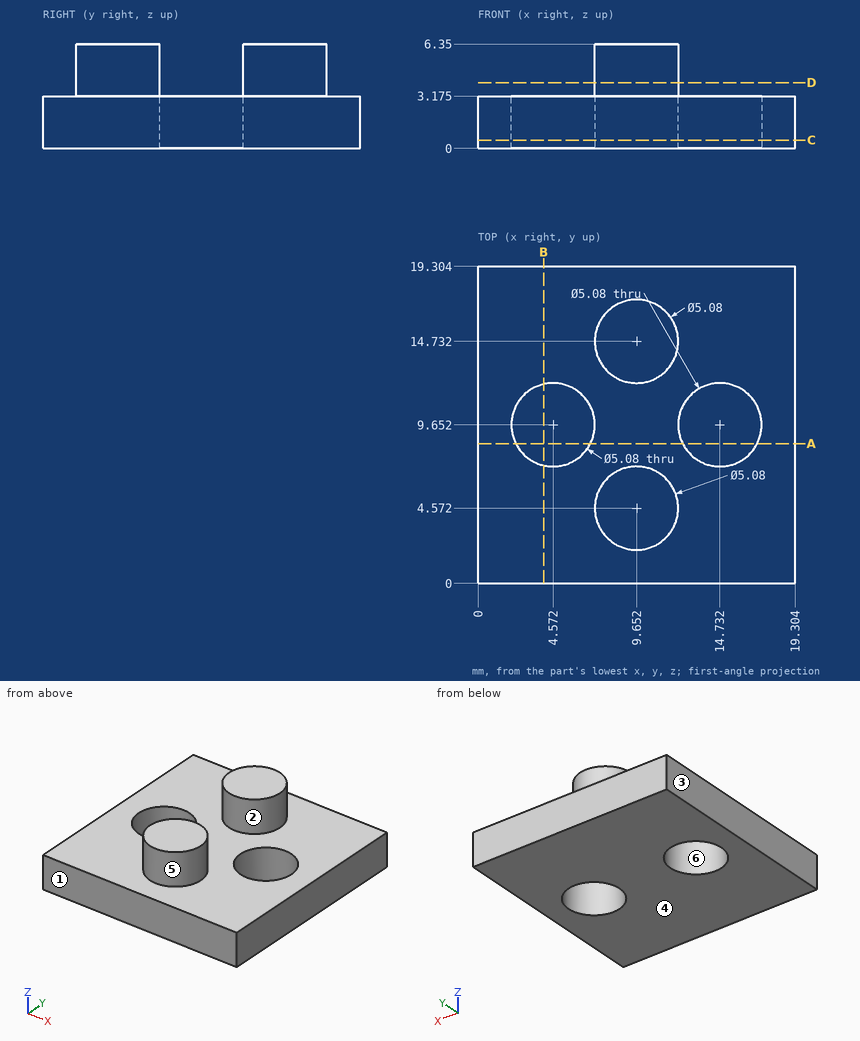
Geometry: see drawing. Coordinates: mm, zero at the bounding-box minimum. A direction names the side the tool comes from. Give positions to 0.01 mm unless a question says otherwise; leave off trailing zeros. Order: outer loops, then holes, each group sorted by start corner. A loop starts at its lowest first (then second) coordinate and runs counter-clockwise, first axis right, second up. Notation, with made-up numbers: (-2, -10) -> (8, -10) arc R29 cw to (8, 17) -> close; hole circle Ø2 at (41.5, -31.75). An arc over 180 degrees is marked (long way). Write each question's results on one line, items separated by ' | '. Start each with the question number.
1) Set-up query: the marked faces 1 and 2. Return all of +Z, -Z, +X, -X, +Y, -Y with unobstructed straight access to the full face (end or side cutting, diameter ignored); none if empty.
2) Section B-B (x = 4). Return loops of the section in (y, z) (3 decimals), then the cut area to 3 significant figures.
3) Draft query along X for the marked faces 3, 4, 5 and 6. Return one class per face: pulls with the +X half, pulls with the -X half, needs draft (parallel to the pull), parting line crosses it, or undercut.
4) Section A-A (y = 8.5). Return loops of the section in (x, z) (3 decimals), then the cut area to 3 significant figures.
5) Section D-D (z = 4). Return loops of the section in (x, y).
6) Section C-C (z = 0.5). Return loops of the section in (x, y), then the cut area to 3 significant figures.
7) First-contact query: pin 1 (6.5 mm diameter, centred on x = 14.732, y = 9.652, fed in from +Z) (3 decimals). Flat tip, straight axial feed; report the tip coordinate or a pass-through.
8) Line query: line 1 (X direction, y = 10, z = 3); line 2 (X direction, y = 11.75, z = 1); line 3 (Z direction, x = 2, y = 6) (3 decimals). Output: solid intervals per line, ascending. Write a range as from..to.
Calculated:
1) face 1: +Z, -Z, +X, -X, -Y | face 2: +Z
2) outline: (0, 0) -> (7.177, 0) -> (7.177, 3.175) -> (0, 3.175) -> close; (12.127, 0) -> (19.304, 0) -> (19.304, 3.175) -> (12.127, 3.175) -> close | area: 45.6 mm2
3) face 3: pulls with the -X half | face 4: needs draft | face 5: parting line crosses it | face 6: undercut
4) outline: (0, 0) -> (2.308, 0) -> (2.308, 3.175) -> (0, 3.175) -> close; (6.836, 0) -> (12.468, 0) -> (12.468, 3.175) -> (6.836, 3.175) -> close; (16.996, 0) -> (19.304, 0) -> (19.304, 3.175) -> (16.996, 3.175) -> close | area: 32.5 mm2
5) outline: circle Ø5.08 at (9.65, 4.57); circle Ø5.08 at (9.65, 14.73)
6) outline: (0, 0) -> (19.3, 0) -> (19.3, 19.3) -> (0, 19.3) -> close; hole circle Ø5.08 at (4.57, 9.65); hole circle Ø5.08 at (14.73, 9.65) | area: 332 mm2
7) pin 1: z = 3.175
8) line 1: 0..2.06, 7.09..12.22, 17.25..19.3 | line 2: 0..3.14, 6..13.3, 16.16..19.3 | line 3: 0..3.175
